from build123d import *

# Parameters (mm, degrees)
SKETCH_1_W      = 10
SKETCH_1_H      = 3
EXTRUDE_1_DEPTH = 1.5


with BuildPart() as part:
    # 草图1 → 凸台-拉伸1 (new body, symmetric)
    with BuildSketch(Plane.XY):
        with BuildLine():
            Line((-17, 20), (17, 20))
            Line((17, 20), (17, 10))
            Line((17, 10), (20, 10))
            Line((20, 10), (20, 1.224744871))
            ThreePointArc((20, 1.224744871), (17, 0), (20, -1.224744871))
            Line((20, -1.224744871), (20, -10))
            Line((20, -10), (17, -10))
            Line((17, -10), (17, -20))
            Line((17, -20), (-17, -20))
            Line((-17, -20), (-17, -10))
            Line((-17, -10), (-20, -10))
            Line((-20, -10), (-20, -1.224744871))
            ThreePointArc((-20, -1.224744871), (-17, 0), (-20, 1.224744871))
            Line((-20, 1.224744871), (-20, 10))
            Line((-20, 10), (-17, 10))
            Line((-17, 10), (-17, 20))
        make_face()
        with Locations((-5, -16.5)):
            Rectangle(SKETCH_1_W, SKETCH_1_H, mode=Mode.SUBTRACT)
    extrude(amount=EXTRUDE_1_DEPTH, both=True)


solid = part.part
For this review, take the finished solid that the model builds, in its own axes (mm). A direction names the side the tool comes from. Give positions to 0.01 mm unless a question says otherwise; leave off trailing zeros. Loops run counter-clockwise (first coordinate to the right, second up) from the corner with the lowest first, then second, coordinate; pieces in that order, holes last. Notation, with made-up numbers: M 62,-15 L 74,-15 A7 cw 74,-9 Z; hole C -9.75,-4 d7. An arc over 180 degrees is marked long. Put each result on its own line as item: value. Start each with the question number.
(1) Wall thickness on L1, parallel to Y at x = -7.5, z = 0.6; L2, parallel to Y at x = 18.75, z = -0.6; L3, parallel to X at y = -17, z = 0.45: over which ranges is each line inside the solid? List them lowest first.
(2) Machinability: for faces 4 (the flat face through (-17, -15, 0)), 5 (the flat face through (-10, -17, 0)), 6 (the flat face through (-19, 10, 0)), 7 (the flat face through (17, 15, 0)), which of the approach directions +Z, -Z, +X, -X, +Y, -Y give a long, thin tool a straight path to every point of the face, cutting with its end or side? Answer none if there is none.
(3) Add section B-B, the plane x = -4. Write out the cut boundary in (y, z), then the cut area to 3 significant figures.
(4) Add section C-C, the plane x = 18.75. Write out the cut boundary in (y, z).
(5) For pin 1 (1.5 mm diameter, centred on y = -14.5, z = -0.5, fed in from -X); pin 2 (3 mm diameter, centred on x = 18.75, y = 0, fed in from +Z) (3 decimals); pin 3 (1.5 mm diameter, centred on x = -18.5, z = 0.5, fed in from -Y); pin 4 (0.9 mm diameter, centred on y = 13.5, z = 0.5, fed in from +X), all flat-tipped, find the tip position at first contact; note any pin that passes through.
(6) The part is to be moulded in two halves that separate along Y. For faces 1 (the flat face through (19, -10, 0)), 2 (the cylindrical face through (-17, 0, 0)), 3 (the flat face through (-17, 15, 0)), say which applies: +Y half, -Y half, draft (parallel to the pull), parting line (faces both ways), or undercut.
(7) Add section A-A, the plane z = -1. Write out the cut boundary in (x, y), then the cut area to 3 significant figures.
(8) Add section D-D, the plane y = -11. Write out the cut boundary in (x, z), then the cut area to 3 significant figures.
Result:
1. L1: y = -20 to -18, -15 to 20
1. L2: y = -10 to -1.75, 1.75 to 10
1. L3: x = -17 to -10, 0 to 17
2. face 4: +Z, -Z, -X, -Y
2. face 5: +Z, -Z
2. face 6: +Z, -Z, -X, +Y
2. face 7: +Z, -Z, +X, +Y
3. outline: M -20,-1.5 L -18,-1.5 L -18,1.5 L -20,1.5 Z; M -15,-1.5 L 20,-1.5 L 20,1.5 L -15,1.5 Z
3. area: 111 mm^2
4. outline: M -10,-1.5 L -1.75,-1.5 L -1.75,1.5 L -10,1.5 Z; M 1.75,-1.5 L 10,-1.5 L 10,1.5 L 1.75,1.5 Z
5. pin 1: stops at x = -17
5. pin 2: passes through
5. pin 3: stops at y = -10
5. pin 4: stops at x = 17
6. face 1: -Y half
6. face 2: undercut
6. face 3: draft
7. outline: M -20,-10 L -17,-10 L -17,-20 L 17,-20 L 17,-10 L 20,-10 L 20,-1.22 A1.75 cw long 20,1.22 L 20,10 L 17,10 L 17,20 L -17,20 L -17,10 L -20,10 L -20,1.22 A1.75 cw long -20,-1.22 Z; hole M -10,-18 L 0,-18 L 0,-15 L -10,-15 Z
7. area: 1,430 mm^2
8. outline: M -17,-1.5 L 17,-1.5 L 17,1.5 L -17,1.5 Z
8. area: 102 mm^2
